from build123d import *

# Parameters (mm, degrees)
SKETCH_1_W          = 42
SKETCH_1_H          = 7.4
EXTRUDE_1_DEPTH     = 2.5
SKETCH_2_R          = 1.5
EXTRUDE_2_DEPTH     = 3.5
SKETCH_3_W          = 29
SKETCH_3_H          = 7.4
CUT_EXTRUDE_1_DEPTH = 0.5
SKETCH_4_W          = 13
SKETCH_4_H          = 0.7
CUT_EXTRUDE_2_DEPTH = 0.5
CUT_EXTRUDE_3_REACH = 44.834
SKETCH_5_W          = 42
SKETCH_5_H          = 0.5
FILLET_1_R          = 1
FILLET_2_R          = 1


with BuildPart() as part:
    # 草图1 → 凸台-拉伸1 (new body)
    with BuildSketch(Plane(origin=(0, 0, 0), x_dir=(1, 0, 0), z_dir=(0, 1, 0))):
        with Locations((21, 3.7)):
            Rectangle(SKETCH_1_W, SKETCH_1_H)
    extrude(amount=EXTRUDE_1_DEPTH)

    # 草图2 → 凸台-拉伸2 (add)
    with BuildSketch(Plane(origin=(0, 2.5, 0), x_dir=(1, 0, 0), z_dir=(0, 1, 0))):
        with Locations(Location((32, 3.4, 0), (0, 0, 90))):
            Circle(SKETCH_2_R)
    extrude(amount=EXTRUDE_2_DEPTH)

    # 草图3 → 切除-拉伸1 (cut)
    with BuildSketch(Plane(origin=(0, 2.5, 0), x_dir=(1, 0, 0), z_dir=(0, 1, 0))):
        with Locations((14.5, 3.7)):
            Rectangle(SKETCH_3_W, SKETCH_3_H)
    extrude(amount=-CUT_EXTRUDE_1_DEPTH, mode=Mode.SUBTRACT)

    # 草图4 → 切除-拉伸2 (cut)
    with BuildSketch(Plane(origin=(0, 2.5, 0), x_dir=(1, 0, 0), z_dir=(0, 1, 0))):
        with Locations((35.5, 7.05)):
            Rectangle(SKETCH_4_W, SKETCH_4_H)
        with Locations((35.5, 0.35)):
            Rectangle(SKETCH_4_W, SKETCH_4_H)
    extrude(amount=-CUT_EXTRUDE_2_DEPTH, mode=Mode.SUBTRACT)

    # 草图5 → 切除-拉伸3 (cut, up to next)
    with BuildSketch(Plane(origin=(0, 2, 0), x_dir=(1, 0, 0), z_dir=(0, 1, 0)), mode=Mode.PRIVATE) as cut_extrude_3_sk1:
        with Locations((21, 0.25)):
            Rectangle(SKETCH_5_W, SKETCH_5_H)
    cut_extrude_3_tool1 = extrude(cut_extrude_3_sk1.sketch, amount=-CUT_EXTRUDE_3_REACH, mode=Mode.PRIVATE) & part.part
    add(cut_extrude_3_tool1.solids().sort_by_distance((21, 2, -0.25))[0], mode=Mode.SUBTRACT)

    # 圆角1
    fillet_1_edges = [part.edges().sort_by_distance(p)[0] for p in [
        (0, 1, -7.4),
        (29, 2.25, -6.7),
        (42, 2.25, -6.7),
        (29, 2.25, -0.7),
        (42, 2.25, -0.7),
        (0, 1, -0.5),
    ]]
    fillet(fillet_1_edges, radius=FILLET_1_R)

    # 圆角2
    fillet_2_edges = [part.edges().sort_by_distance(p)[0] for p in [
        (42, 1, -7.4),
        (42, 1, -0.5),
    ]]
    fillet(fillet_2_edges, radius=FILLET_2_R)


solid = part.part
Geometry check sheet. Reference: the model listing, model coordinates, mm. A direction names the side the tool comes from. Give positions to 0.01 mm unless a question says otherwise; leave off trailing zeros. Order: outer loops, then holes, each group sorted by start corner. A loop starts at its lowest first (then second) coordinate and runs counter-clockwise, first axis right, second up.
1. Sectioned sample at C-C (y = 3.15). Record the boundary of the cut face in (x, z), then the cut area to 3 significant figures.
Completed:
outline: circle Ø3 at (32, -3.4)
area: 7.07 mm2
2. Sectioned sample at D-D (x = 12). Record the boundary of the cut face in (y, z).
Completed:
outline: (0, -7.4) - (2, -7.4) - (2, -0.5) - (0, -0.5) - close
3. Sectioned sample at B-B (z = -3.4). Record the boundary of the cut face in (x, y).
Completed:
outline: (0, 0) - (42, 0) - (42, 2.5) - (33.5, 2.5) - (33.5, 6) - (30.5, 6) - (30.5, 2.5) - (29, 2.5) - (29, 2) - (0, 2) - close
4. Scan lines: line 1 (X direction, y = 2.35, z = -4.5); line 2 (Y direction, x = 19.5, z = -1.25); line 3 (X direction, y = 3.25, z = -2.5). Record each from-to range of solid material in increasing order.
Completed:
line 1: x = 29 to 42
line 2: y = 0 to 2
line 3: x = 30.8 to 33.2
5. Access from +Z, -Z, +X, -X, +Y, -Y to the whole of each face (thin tool, end or side, straight path). Record for faces 1 (the face through (0, 1, -4)), 2 (the face through (41.715, 2.246, -1.001)), 3 (the face through (41.715, 2.246, -6.399)), 4 (the face through (29.285, 2.246, -1.001)), 5 (the face through (32, 6, -3)).
Completed:
face 1: +Z, -Z, -X, +Y, -Y
face 2: +Z, +X, +Y
face 3: -Z, +X, +Y
face 4: +Z, -X, +Y
face 5: +Z, -Z, +X, -X, +Y
6. Sectioned sample at A-A (x = 35). Record the boundary of the cut face in (y, z), then the cut area to 3 significant figures.
Completed:
outline: (0, -7.4) - (2, -7.4) - (2, -6.7) - (2.5, -6.7) - (2.5, -0.7) - (2, -0.7) - (2, -0.5) - (0, -0.5) - close
area: 16.8 mm2
7. Draft check along X on faces 6 (the face through (16, 2, -4)), 7 (the face through (29.301, 2.246, -6.415)), 8 (the face through (42, 1, -4)), 9 (the face through (30.735, 4.226, -4.206)). Enter one of: pulls with the +X half, pulls with the -X half, needs draft (parallel to the pull), parting line crosses it, or undercut.
Completed:
face 6: needs draft
face 7: pulls with the -X half
face 8: pulls with the +X half
face 9: parting line crosses it
